```python
from build123d import *

# Parameters (mm, degrees)
CROQUIS1_W              = 50.8
CROQUIS1_H              = 6.31
SALIENTE_EXTRUIR1_DEPTH = 228.75
CROQUIS2_W              = 50.8
CROQUIS2_H              = 6.31
SALIENTE_EXTRUIR2_DEPTH = 535.27
CROQUIS3_W              = 50.8
CROQUIS3_H              = 6.31
SALIENTE_EXTRUIR3_DEPTH = 552.5
CROQUIS4_W              = 50.8
CROQUIS4_H              = 6.31
SALIENTE_EXTRUIR4_DEPTH = 324.39
CROQUIS5_W              = 50.8
CROQUIS5_H              = 6.31
SALIENTE_EXTRUIR5_DEPTH = 50.8
CROQUIS7_R              = 5
CORTAR_EXTRUIR2_DEPTH   = 415.8
CROQUIS8_R              = 6.5
CORTAR_EXTRUIR3_DEPTH   = 10
CROQUIS9_R              = 5
CORTAR_EXTRUIR4_DEPTH   = 35


with BuildPart() as part:
    # Croquis1 → Saliente-Extruir1 (new body)
    with BuildSketch(Plane.XY):
        Rectangle(CROQUIS1_W, CROQUIS1_H)
    extrude(amount=SALIENTE_EXTRUIR1_DEPTH)

    # Croquis2 → Saliente-Extruir2 (add)
    with BuildSketch(Plane.XZ.offset(3.155)):
        with Locations((0, 225.595)):
            Rectangle(CROQUIS2_W, CROQUIS2_H)
    extrude(amount=SALIENTE_EXTRUIR2_DEPTH)

    # Croquis3 → Saliente-Extruir3 (add)
    with BuildSketch(Plane.XY.offset(228.75)):
        with Locations((0, -535.27)):
            Rectangle(CROQUIS3_W, CROQUIS3_H)
    extrude(amount=SALIENTE_EXTRUIR3_DEPTH)

    # Croquis4 → Saliente-Extruir4 (add)
    with BuildSketch(Plane(origin=(0, -532.115, 0), x_dir=(1, 0, 0), z_dir=(0, 1, 0))):
        with Locations((0, -778.095)):
            Rectangle(CROQUIS4_W, CROQUIS4_H)
    extrude(amount=SALIENTE_EXTRUIR4_DEPTH)

    # Croquis5 → Saliente-Extruir5 (add)
    with BuildSketch(Plane(origin=(0, 3.155, 0), x_dir=(1, 0, 0), z_dir=(0, 1, 0))):
        with Locations((0, -3.155)):
            Rectangle(CROQUIS5_W, CROQUIS5_H)
    extrude(amount=-SALIENTE_EXTRUIR5_DEPTH)

    # Croquis7 → Cortar-Extruir2 (cut)
    with BuildSketch(Plane.XY.offset(6.31)):
        with Locations((0, -22.245)):
            Circle(CROQUIS7_R)
    extrude(amount=-CORTAR_EXTRUIR2_DEPTH, mode=Mode.SUBTRACT)

    # Croquis8 → Cortar-Extruir3 (cut)
    with BuildSketch(Plane.XY.offset(781.25)):
        with Locations((0, -224.225)):
            Circle(CROQUIS8_R)
        with Locations((0, -255.225)):
            Circle(CROQUIS8_R)
    extrude(amount=-CORTAR_EXTRUIR3_DEPTH, mode=Mode.SUBTRACT)

    # Croquis9 → Cortar-Extruir4 (cut)
    with BuildSketch(Plane.XY.offset(781.25)):
        with Locations((0, -451.925)):
            Circle(CROQUIS9_R)
    extrude(amount=-CORTAR_EXTRUIR4_DEPTH, mode=Mode.SUBTRACT)


solid = part.part
```
Can you work these out from the model? Positions are in its coordinate system, mm. A direction names the side the tool comes from. Give positions to 0.01 mm unless a question says otherwise; leave off trailing zeros. Loops run counter-clockwise (first coordinate to the right, second up) from the corner with the lowest first, then second, coordinate; pieces in that order, holes last. Notation, with made-up numbers: M -26,-32 L -4,-32 A24 cw -4,-16 Z; hole C 67.5,39 d8. An arc over 180 degrees is marked long. One line per item, written item: value.
(1) Which directions (+Z, -Z, +X, -X, +Y, -Y) give clear straight access to the entire face, cutting with the end or side of a thin tool? Please do faces 1 (the face through (0, -372, 774.94)), 2 (the face through (0, -375, 781.25)), 3 (the face through (0, -30, 6.31)).
Returned:
face 1: +X, -X, +Y
face 2: +Z, +X, -X, +Y, -Y
face 3: +X, -X, -Y
(2) We'd pull the mould along Z, two halves only. Please class faces 4 (the face through (0, -532.115, 498)), 5 (the face through (0, -261, 228.75)), 6 (the face through (5.3, -21.9, 0)), 7 (the face through (0, -538.425, 498)): released by +Z, released by -Z, zero draft, split by the parting line, or undercut.
Returned:
face 4: undercut
face 5: undercut
face 6: released by -Z
face 7: zero draft
(3) I need wall thicknesses on line 1 (Y direction, x = 0, z = 777.25) (3 decimals); line 2 (Z direction, x = -4.5, y = -446); line 3 (Y direction, x = -6, z = 202) (3 decimals). Which ranges of each line are inside material? Lowest first, please.
Returned:
line 1: -538.425 to -456.925, -446.925 to -261.725, -248.725 to -230.725, -217.725 to -207.725
line 2: 222.44 to 228.75, 774.94 to 781.25
line 3: -3.155 to 3.155
(4) Will these pins go through, and if not, where does the flat tip stop? pin 1 (3 mm diameter, centred on x = 1, z = 372, fed in from +Y) (3 decimals); pin 2 (5 mm diameter, centred on x = 9, y = -259.5, fed in from -Z); pin 3 (7 mm diameter, centred on x = 5.5, z = 777, fed in from +Y) (3 decimals).
Returned:
pin 1: y = -532.115
pin 2: z = 222.44
pin 3: y = -207.725
(5) Suppose I cut it at A-A on y = -302. List the corners of the cut face in (x, z) for me, plus the area to 3 significant figures.
Returned:
outline: M -25.4,222.44 L 25.4,222.44 L 25.4,228.75 L -25.4,228.75 Z; M -25.4,774.94 L 25.4,774.94 L 25.4,781.25 L -25.4,781.25 Z
area: 641 mm^2
(6) Suppose I cut it at C-C on y = -90. List the corners of the cut face in (x, z) for me.
Returned:
outline: M -25.4,222.44 L 25.4,222.44 L 25.4,228.75 L -25.4,228.75 Z
(7) Suppose I cut it at B-B on z = 156. List the corners of the cut face in (x, y) for me (3 decimals), plus the area to 3 significant figures.
Returned:
outline: M -25.4,-3.155 L 25.4,-3.155 L 25.4,3.155 L -25.4,3.155 Z
area: 321 mm^2
